```python
from build123d import *

# Parameters (mm, degrees)
SKETCH1_W               = 50
SKETCH1_H               = 65
BOSS_EXTRUDE1_DEPTH     = 10
CUT_EXTRUDE1_DEPTH      = 43.20485754
CUT_EXTRUDE1_DEPTH_BACK = 43.20485754
SKETCH6_R               = 2
SKETCH6_R_2             = 2.25
SKETCH7_R               = 2
CUT_EXTRUDE2_DEPTH      = 43.20485754
SKETCH8_W               = 2.7
SKETCH8_H               = 7.5
SKETCH8_W_2             = 7.5
SKETCH8_H_2             = 2.7
CUT_EXTRUDE3_DEPTH      = 8.75


with BuildPart() as part:
    # Sketch1 → Boss-Extrude1 (new body)
    with BuildSketch(Plane(origin=(0, 0, 0), x_dir=(1, 0, 0), z_dir=(0, 1, 0))):
        Rectangle(SKETCH1_W, SKETCH1_H)
        with BuildLine():
            Line((-15, 0), (-15, -20))
            Line((-15, -20), (15, -20))
            Line((15, -20), (15, 0))
            ThreePointArc((15, 0), (0, 15), (-15, 0))
        make_face(mode=Mode.SUBTRACT)
    extrude(amount=BOSS_EXTRUDE1_DEPTH)

    # Sketch6 → Cut-Extrude1 (cut, two sides: drawn at the far end of the back side and taken through both)
    with BuildSketch(Plane(origin=(0, 0, 0), x_dir=(0, 0, -1), z_dir=(1, 0, 0)).offset(-CUT_EXTRUDE1_DEPTH_BACK)):
        with Locations((-7.5, 5)):
            Circle(SKETCH6_R)
        with Locations((26.5, 5)):
            Circle(SKETCH6_R_2)
    extrude(amount=CUT_EXTRUDE1_DEPTH + CUT_EXTRUDE1_DEPTH_BACK, mode=Mode.SUBTRACT)

    # Sketch7 → Cut-Extrude2 (cut, through all)
    with BuildSketch(Plane.XY):
        with Locations(Location((0, 5, 0), (0, 0, 180))):
            Circle(SKETCH7_R)
    extrude(amount=CUT_EXTRUDE2_DEPTH, mode=Mode.SUBTRACT)

    # Sketch8 → Cut-Extrude3 (cut)
    with BuildSketch(Plane(origin=(0, 0, 0), x_dir=(1, 0, 0), z_dir=(0, 1, 0))):
        with Locations((20, -7.5)):
            Rectangle(SKETCH8_W, SKETCH8_H)
        with Locations((-20, -7.5)):
            Rectangle(SKETCH8_W, SKETCH8_H)
        with Locations((0, -26.25)):
            Rectangle(SKETCH8_W_2, SKETCH8_H_2)
    extrude(amount=CUT_EXTRUDE3_DEPTH, mode=Mode.SUBTRACT)


solid = part.part
```
Model file for the job. Use its own axes, mm. A direction names the side the tool comes from. Round coordinates to 2 decimals unless told otherwise and drop trailing zeros. Order: outer loops, then holes, each group sorted by start corner. A loop starts at its lowest first (then second) coordinate and runs counter-clockwise, first axis right, second up. Notation, with made-up numbers: (13, -21) -> (64, -21) arc R26 cw to (64, 14) -> close; hole circle Ø11 at (-2, -30). An arc over 180 degrees is marked (long way). Use one line per item in the form item = value.
Item 1: Drill centre lines: line 1 (Z direction, x = -16.35, y = 5); line 2 (Z direction, x = -21, y = 7.5); line 3 (Y direction, x = 16.5, z = 7.5). Where is each one in solid material? Low to high.
Returned:
line_1 = -32.5 to -28.75, -24.25 to 5.5, 9.5 to 32.5
line_2 = -32.5 to 3.75, 11.25 to 32.5
line_3 = 0 to 3, 7 to 10
Item 2: Tool access for faces 1 (the face through (0, 7, 30)), 2 (the face through (-23.201, 5.088, 9.498)), 3 (the face through (-20, 8.75, 7)): list every direction of +Z, -Z, +X, -X, +Y, -Y with a clear straight run to the whole face (end or side of a thin tool).
Returned:
face_1 = +Z
face_2 = +X, -X
face_3 = -Y
Item 3: Cut at A-A, the plane x = 0. Write the cut outline in (y, z), and give its area (3 significant figures).
Returned:
outline = (0, -32.5) -> (10, -32.5) -> (10, -15) -> (0, -15) -> close; (0, 20) -> (3, 20) -> (3, 24.9) -> (0, 24.9) -> close; (0, 27.6) -> (3, 27.6) -> (3, 32.5) -> (0, 32.5) -> close; (7, 20) -> (10, 20) -> (10, 32.5) -> (7, 32.5) -> (7, 27.6) -> (8.75, 27.6) -> (8.75, 24.9) -> (7, 24.9) -> close; hole circle Ø4.5 at (5, -26.5)
area = 221 mm^2
Item 4: Pull direction Z, two halves, no side cores. Call faces 4 (the face through (-0.2, 2.7, 20)), 5 (the face through (0, 5, -32.5)), 6 (the face through (-0.3, 2.7, 32.5)): released by +Z, released by -Z, zero draft, split by the parting line, or undercut.
Returned:
face_4 = undercut
face_5 = released by -Z
face_6 = released by +Z
Item 5: Cut at C-C, the plane z = 7.5. Give the number of separate pieces and of enclosed holes in the cut face, and give its area (4 significant figures).
Returned:
separate_pieces = 6
enclosed_holes = 0
area = 94.35 mm^2
Item 6: Flat gauge pin, fed straight in: pin 1 Ø1.4 at (x, z) = (-20.5, 9) entering from -Y. Where does the tip first touch, or does it go through?
Returned:
pin_1 = 8.75
Item 7: Cut at B-B, the plane z = -26.5. Write the cut outline in (x, y), and give its area (3 significant figures).
Returned:
outline = (-25, 0) -> (25, 0) -> (25, 2.75) -> (-25, 2.75) -> close; (-25, 7.25) -> (25, 7.25) -> (25, 10) -> (-25, 10) -> close
area = 275 mm^2
